Input: part model. Units: mm. Frame: model coordinates. A direction names the side the tool comes from. Give positions to 0.01 mm unless a question says otherwise; leave off trailing zeros. Order: outer loops, then holes, each group sorted by start corner. A loop starts at its lowest first (then second) coordinate and runs counter-clockwise, first axis right, second up. Notation, with made-up numbers: (40, 0.25) - (51, 0.25) arc R13 ccw to (51, 10.25) - close; hole circle Ø1 at (8, 11). An arc over 180 degrees is marked (long way). Answer in a Markdown table with one row per item. Add a question column.
from build123d import *

# Parameters (mm, degrees)
BOSS_EXTRUDE1_DEPTH = 15
BOSS_EXTRUDE2_DEPTH = 2.8
SKETCH2_R           = 2.6
CUT_EXTRUDE1_DEPTH  = 22.168136432
SKETCH4_R           = 1.55
CUT_EXTRUDE3_DEPTH  = 2.5
CIRPATTERN1_COUNT   = 3
CHAMFER1_SIZE       = 0.5
CHAMFER2_SIZE       = 0.5
CHAMFER3_SIZE       = 1
CHAMFER4_SIZE       = 0.4


with BuildPart() as part:
    # Sketch1 → Boss-Extrude1 (new body)
    with BuildSketch(Plane.XY):
        Polygon((0, 8.660254038), (-7.5, 4.330127019), (-7.5, -4.330127019), (0, -8.660254038), (7.5, -4.330127019), (7.5, 4.330127019), align=None)
    extrude(amount=BOSS_EXTRUDE1_DEPTH)

    # Sketch3 → Boss-Extrude2 (add)
    with BuildSketch(Plane(origin=(0, 0, 0), x_dir=(-1, 0, 0), z_dir=(0, 0, -1))):
        Polygon((0, 5.773502692), (-5, 2.886751346), (-5, -2.886751346), (0, -5.773502692), (5, -2.886751346), (5, 2.886751346), align=None)
    extrude(amount=BOSS_EXTRUDE2_DEPTH)

    # Sketch2 → Cut-Extrude1 (cut, through all)
    with BuildSketch(Plane.XY.offset(15)):
        Circle(SKETCH2_R)
    extrude(amount=-CUT_EXTRUDE1_DEPTH, mode=Mode.SUBTRACT)

    # Sketch4 → Cut-Extrude3 (cut)
    with BuildSketch(Plane(origin=(3.75, 6.495190528, 0), x_dir=(0.8660254037844417, -0.4999999999999949, 0), z_dir=(0.4999999999999949, 0.8660254037844417, 0))):
        with Locations(Location((0, -10, 0), (0, 0, 180))):
            Circle(SKETCH4_R)
    cut_extrude3 = extrude(amount=-CUT_EXTRUDE3_DEPTH, mode=Mode.SUBTRACT)

    # CirPattern1: Cut-Extrude3 ×3 about axis
    cirpattern1_axis = Axis((0, 0, 0), (0, 0, 1))
    for i in range(1, CIRPATTERN1_COUNT):
        add(cut_extrude3.rotate(cirpattern1_axis, i * 360 / CIRPATTERN1_COUNT), mode=Mode.SUBTRACT)

    # Chamfer1
    chamfer1_edges = [part.edges().sort_by_distance(p)[0] for p in [
        (-7.5, 0, 15),
        (-3.75, -6.495190528, 15),
        (3.75, -6.495190528, 15),
        (7.5, 0, 15),
        (-2.6, 0, 15),
        (3.75, 6.495190528, 15),
        (-3.75, 6.495190528, 15),
    ]]
    chamfer(chamfer1_edges, length=CHAMFER1_SIZE)

    # Chamfer2
    chamfer2_edges = [part.edges().sort_by_distance(p)[0] for p in [
        (5.092339376, 5.720190528, 10),
        (-7.5, 1.55, 10),
        (2.407660624, -7.270190528, 10),
    ]]
    chamfer(chamfer2_edges, length=CHAMFER2_SIZE)

    # Chamfer3
    chamfer3_edges = [part.edges().sort_by_distance(p)[0] for p in [
        (-2.6, 0, -2.8),
    ]]
    chamfer(chamfer3_edges, length=CHAMFER3_SIZE)

    # Chamfer4
    chamfer4_edges = [part.edges().sort_by_distance(p)[0] for p in [
        (-2.5, 4.330127019, -2.8),
        (2.5, 4.330127019, -2.8),
        (5, 0, -2.8),
        (2.5, -4.330127019, -2.8),
        (-2.5, -4.330127019, -2.8),
        (-5, 0, -2.8),
    ]]
    chamfer(chamfer4_edges, length=CHAMFER4_SIZE)


solid = part.part
Q1. Section A-A, the plane y = 0. Return loops of the section in (x, z).
Q2. Section B-B, the plane z = -1.5. Return loops of the section in (x, y), then the cut area to 3 significant figures.
Q3. Section C-C, the plane z = 5. Return loops of the section in (x, y), then the cut area to 3 significant figures.
Q4. Line query: probe 1 along Y at (x, z) = (1.75, 10.5); probe 2 along Y at (x, z) = (-3, -1); probe 3 along Y at (x, z) = (1.5, 3.25). Output: solid intervals per line, ascending.
Q5. Access query for faces 5 (the flat face through (2.48, -4.34, 10.02)), 6 (the flat face through (2.535, -4.31, -1.183)), 7 (the flat face through (5, 0, -1)), 8 (the flat face through (-5, 0, 10)). Directions: +Z, -Z, +X, -X, +Y, -Y. A direction counts if a zero-diameter tool reaches every point of the face in a straight line with its end or side. Return the directions, or none.
Q6. Contact query for flat-ended pins moving along their axis: P1, Ø0.9, axis at y = 0.5, z = 10.5, coming from the -X side; P2, Ø2, axis at x = 5.5, z = -0.5, coming from the +Y side; P3, Ø3, axis at x = 4, z = 5, coming from the +Y side; P4, Ø4.5, axis at x = 0, y = 0, coming from the +Z side. Output: stop coordinate, or through.
Q7. Pull-direction query (Y, two-part tool) for faces 1 (the flat face through (-3.802, -6.465, 7.148)), 2 (the cylindrical face through (3.298, 5.04, 8.487)), 3 (the cylindrical face through (-0.338, 2.578, 6.464)), 4 (the flat face through (-5, 0, -1)); classes: +Y half, -Y half, draft (parallel to the pull), parting line (faces both ways), or undercut.
Computed:
| question | item | result |
|---|---|---|
| 1 | outline | (-7.5, 0) - (-5, 0) - (-5, -2.4) - (-4.6, -2.8) - (-3.6, -2.8) - (-2.6, -1.8) - (-2.6, 14.5) - (-3.1, 15) - (-7, 15) - (-7.5, 14.5) - (-7.5, 12.05) - (-7, 11.55) - (-5, 11.55) - (-5, 8.45) - (-7, 8.45) - (-7.5, 7.95) - close; (2.6, -1.8) - (3.6, -2.8) - (4.6, -2.8) - (5, -2.4) - (5, 0) - (7.5, 0) - (7.5, 14.5) - (7, 15) - (3.1, 15) - (2.6, 14.5) - close |
| 2 | outline | (-5, -2.89) - (0, -5.77) - (5, -2.89) - (5, 2.89) - (0, 5.77) - (-5, 2.89) - close; hole circle Ø5.2 at (0, 0) |
| 2 | area | 65.4 mm^2 |
| 3 | outline | (-7.5, -4.33) - (0, -8.66) - (7.5, -4.33) - (7.5, 4.33) - (0, 8.66) - (-7.5, 4.33) - close; hole circle Ø5.2 at (0, 0) |
| 3 | area | 174 mm^2 |
| 4 | probe 1 | y = -7.65 to -5.97, -4.76 to -1.92, 1.92 to 4.76, 5.97 to 7.65 |
| 4 | probe 2 | y = -4.04 to 4.04 |
| 4 | probe 3 | y = -7.79 to -2.12, 2.12 to 7.79 |
| 5 | face 5 | none |
| 5 | face 6 | -Z, +X, -Y |
| 5 | face 7 | -Z, +X, +Y, -Y |
| 5 | face 8 | -X |
| 6 | P1 | stops at x = -5 |
| 6 | P2 | stops at y = 5.98 |
| 6 | P3 | stops at y = 7.22 |
| 6 | P4 | passes through |
| 7 | face 1 | -Y half |
| 7 | face 2 | undercut |
| 7 | face 3 | undercut |
| 7 | face 4 | draft |
